from build123d import *

# Parameters (mm, degrees)
F1_DEPTH = 38.1
F2_W     = 12.7
F2_H     = 12.7
F3_DEPTH = 25.4
F4_W     = 12.7
F4_H     = 6.35
F5_DEPTH = 25.4


# Not quite as in the source:
# - a feature names something its author has since deleted; it is built from what else it names


with BuildPart() as f1:
    # F0 (on Right) → F1 (new body)
    with BuildSketch(Plane.YZ):
        Polygon((-25.4, 0), (0, 0), (0, 31.75), (-12.7, 31.75), (-12.7, 12.7), (-25.4, 12.7), align=None)
    extrude(amount=F1_DEPTH)

    # F2 (on Top) → F3 (join)
    with BuildSketch(Plane.XY):
        with Locations((19.05, -6.35)):
            Rectangle(F2_W, F2_H)
    extrude(amount=F3_DEPTH)

    # F4 (on Front) → F5 (cut)
    with BuildSketch(Plane.XZ):
        with Locations((19.05, 28.8461486514)):
            Rectangle(F4_W, F4_H)
    extrude(amount=F5_DEPTH, mode=Mode.SUBTRACT)


solid = f1.part
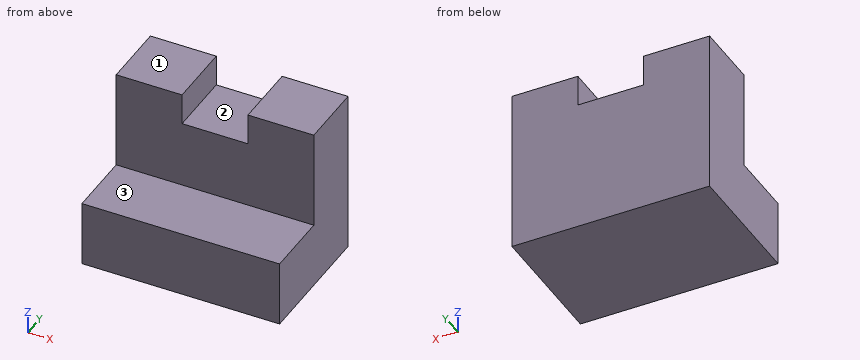
Design review of the part built by this model. Coordinates are the model's own, in mm. Face numbers are marked on the shaded views. A direction names the side the tool comes from. Coordinates: 2 decimals unless noted, no trailing zeros. Order: outer loops, then holes, each group sorted by start corner. A loop starts at its lowest first (then second) coordinate and runs counter-clockwise, first axis right, second up. Notation, with made-up numbers: M 75,8 L 118,8 A15 cw 118,18 Z; hole C -4.5,-36 d11. An arc over 180 degrees is marked long. Use a Markdown table: item, result.
(1) Add section B-B (x = 9.5). Give the boundary of the cut face in (y, z), then the cut area to 3 significant figures.
Worked answers:
| item | result |
|---|---|
| outline | M -25.4,0 L 0,0 L 0,31.75 L -12.7,31.75 L -12.7,12.7 L -25.4,12.7 Z |
| area | 565 mm2 |
(2) Add section D-D (y = -20). Give the boundary of the cut face in (x, z).
Worked answers:
| item | result |
|---|---|
| outline | M 0,0 L 38.1,0 L 38.1,12.7 L 0,12.7 Z |
(3) Add section C-C (z = 21). Give the boundary of the cut face in (x, y), then the cut area to 3 significant figures.
Worked answers:
| item | result |
|---|---|
| outline | M 0,-12.7 L 38.1,-12.7 L 38.1,0 L 0,0 Z |
| area | 484 mm2 |
(4) For P1, Ø10, axis at x = 26.5, z = 23, coming from the -Y side, flat-tipped, find the tip position at first contact; note if it passes through.
Worked answers:
| item | result |
|---|---|
| P1 | stops at y = -12.7 |
(5) Add section A-A (y = -11.75). Give the boundary of the cut face in (x, z).
Worked answers:
| item | result |
|---|---|
| outline | M 0,0 L 38.1,0 L 38.1,31.75 L 25.4,31.75 L 25.4,25.67 L 12.7,25.67 L 12.7,31.75 L 0,31.75 Z |
(6) For the marked faces 1, 2 and 3, list the 3-axis set-ups (+Z, -Z, +X, -X, +Y, -Y) from which the entire face can be reached by the end or side of a thin tool; tool diameter is ignored.
Worked answers:
| item | result |
|---|---|
| face 1 | +Z, +X, -X, +Y, -Y |
| face 2 | +Z, +Y, -Y |
| face 3 | +Z, +X, -X, -Y |
(7) Wall thickness on probe 1 along Y at (x, z) = (26, 21); probe 2 along Z at (x, y) = (13.5, -2.25); probe 3 along Z at (x, y) = (29, -22.25): over which ranges is each line inside the solid? List them lowest first.
Worked answers:
| item | result |
|---|---|
| probe 1 | y = -12.7 to 0 |
| probe 2 | z = 0 to 25.67 |
| probe 3 | z = 0 to 12.7 |
